Build history of the part. All positions in model axes, mm. Face numbers are marked on the shaded views. Coordinates: 2 decimals unless noted, no trailing zeros. Order: outer loops, then holes, each group sorted by start corner. A loop starts at its lowest first (then second) coordinate and runs counter-clockwise, first axis right, second up. Notation, with made-up numbers: (-35, -18.5) - (-20, -18.5) arc R24 ccw to (-20, 15.5) - close; hole circle Ø9 at (30, -29). An arc over 180 degrees is marked (long way). One line per item, written item: value.
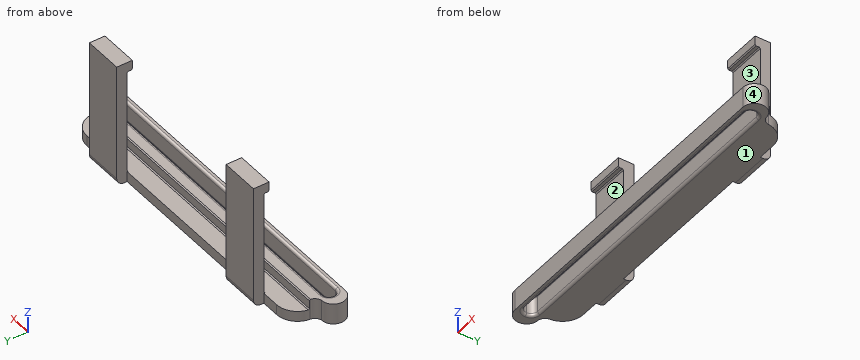
from build123d import *

# Parameters (mm, degrees)
F1_DEPTH    = 8
F2_DEPTH    = 8
F3_DEPTH    = 4
F0_W        = 15
F0_H        = 4
F4_DEPTH    = 48
F5_W        = 15
F5_H        = 3.75
F6_DEPTH    = 2
F7_T1_DEPTH = 43.7732905232
F8_R        = 1
F9_R        = 1
F10_R       = 3
F11_SIZE    = 0.4


# Not quite as in the source:
# - a fillet or chamfer that OpenCascade refuses, or shapes differently, is made with other operations: its cross-section is extruded or revolved along the edge and cut away or added


with BuildPart() as f1:
    # F0 (on Top) → F1 (new body)
    with BuildSketch(Plane.XY):
        with BuildLine():
            Line((60, -5), (-60, -5))
            ThreePointArc((-60, -5), (-61.767766953, -4.267766953), (-62.5, -2.5))
            Line((-62.5, -2.5), (-62.5, -7))
            Line((-62.5, -7), (62.5, -7))
            Line((62.5, -7), (62.5, -2.5))
            ThreePointArc((62.5, -2.5), (61.767766953, -4.267766953), (60, -5))
        make_face()
        with BuildLine():
            Line((62.5, 2), (62.5, -2.5))
            Line((62.5, -2.5), (62.5, -7))
            ThreePointArc((62.5, -7), (67, -2.5), (62.5, 2))
        make_face()
        with BuildLine():
            Line((-62.5, -7), (-62.5, -2.5))
            Line((-62.5, -2.5), (-62.5, 2))
            ThreePointArc((-62.5, 2), (-67, -2.5), (-62.5, -7))
        make_face()
        with BuildLine():
            ThreePointArc((-62.5, -2.5), (-61.767766953, -0.732233047), (-60, 0))
            Line((-60, 0), (60, 0))
            ThreePointArc((60, 0), (61.767766953, -0.732233047), (62.5, -2.5))
            Line((62.5, -2.5), (62.5, 2))
            Line((62.5, 2), (-62.5, 2))
            Line((-62.5, 2), (-62.5, -2.5))
        make_face()
    extrude(amount=F1_DEPTH)

    # F0 (on Top) → F2 (join)
    with BuildSketch(Plane.XY):
        with BuildLine():
            ThreePointArc((-60, 5), (-60.7069250972, 3.047437581), (-62.5, 2))
            Line((-62.5, 2), (62.5, 2))
            ThreePointArc((62.5, 2), (60.7069250972, 3.047437581), (60, 5))
            Line((60, 5), (-60, 5))
        make_face()
    extrude(amount=F2_DEPTH)

    # F0 (on Top) → F3 (join)
    with BuildSketch(Plane.XY):
        Polygon((-60, 12), (-60, 5), (60, 5), (60, 12), (45, 12), (30, 12), (-30, 12), (-45, 12), align=None)
    extrude(amount=F3_DEPTH)

    # F0 (on Top) → F4 (join)
    with BuildSketch(Plane.XY):
        with Locations((-37.5, 14)):
            Rectangle(F0_W, F0_H)
        with Locations((37.5, 14)):
            Rectangle(F0_W, F0_H)
    extrude(amount=F4_DEPTH)

    # F5 (on face) → F6 (join)
    with BuildSketch(Plane.XZ.offset(-12)):
        with Locations((-37.5, 46.125)):
            Rectangle(F5_W, F5_H)
        with Locations((37.5, 46.125)):
            Rectangle(F5_W, F5_H)
    extrude(amount=F6_DEPTH)

    # F7: fillet of radius 8 on 2 edges, made by hand

    # F7_s2 → F7_t1 (cut)
    with BuildSketch(Plane.XY.offset(-19.8866452616)):
        with BuildLine():
            ThreePointArc((52.0453418954, 12), (57.4401609283, 9.9072775118), (60.0125151838, 4.7239819005))
            Line((60.0125151838, 4.7239819005), (60.8092325126, 4.7963800905))
            ThreePointArc((60.8092325126, 4.7963800905), (60.8, 5), (60.8, 12))
            Line((60.8, 12), (60, 12.8))
            Line((60, 12.8), (52.0453418954, 12.8))
            Line((52.0453418954, 12.8), (52.0453418954, 12))
        make_face()
        with BuildLine():
            ThreePointArc((-60.0125151838, 4.7239819005), (-57.4401609283, 9.9072775118), (-52.0453418954, 12))
            Line((-52.0453418954, 12), (-52.0453418954, 12.8))
            Line((-52.0453418954, 12.8), (-60, 12.8))
            Line((-60, 12.8), (-60.8, 12))
            ThreePointArc((-60.8, 12), (-60.8, 5), (-60.8092325126, 4.7963800905))
            Line((-60.8092325126, 4.7963800905), (-60.0125151838, 4.7239819005))
        make_face()
    extrude(amount=F7_T1_DEPTH, mode=Mode.SUBTRACT)

    # F8
    f8_edges = [f1.edges().sort_by_distance(p)[0] for p in [
        (0, 0, 8),
    ]]
    fillet(f8_edges, radius=F8_R)

    # F9
    f9_edges = [f1.edges().sort_by_distance(p)[0] for p in [
        (0, -5, 0),
        (62.5, -2.5, 0),
        (-62.5, -2.5, 0),
        (0, 0, 0),
    ]]
    fillet(f9_edges, radius=F9_R)

    # F10
    f10_edges = [f1.edges().sort_by_distance(p)[0] for p in [
        (-37.5, 16, 0),
        (37.5, 16, 0),
    ]]
    fillet(f10_edges, radius=F10_R)

    # F11
    f11_edges = [f1.edges().sort_by_distance(p)[0] for p in [
        (0, 5, 4),
        (-37.5, 12, 4),
        (37.5, 12, 4),
        (0, 5, 8),
        (37.5, 12, 44.25),
        (-37.5, 12, 44.25),
        (-37.5, 10, 44.25),
        (37.5, 10, 44.25),
    ]]
    chamfer(f11_edges, length=F11_SIZE)


solid = f1.part
1. Two-plate mould, pull along Z, no slides. Class the marked faces 1, 2, 3 and 4: pulls with the +Z half, pulls with the -Z half, needs draft (parallel to the pull), parting line crosses it, or undercut.
Values found:
face 1: pulls with the -Z half
face 2: undercut
face 3: undercut
face 4: needs draft
2. Band-saw the part on B-B, the plane z = 39.5. Give the cut face in (x, y).
Values found:
outline: (-45, 12) - (-30, 12) - (-30, 16) - (-45, 16) - close; (30, 12) - (45, 12) - (45, 16) - (30, 16) - close
3. Probe line 1 along X through (y, z) = (15, 44.5); line 2 along Y through (x, z) = (12, 3.5); line 3 along Y through (x, z) = (-50, 6). List the from-to ranges inside material, lowest first.
Values found:
line 1: x = -45 to -30, 30 to 45
line 2: y = -7 to -5, 0 to 12
line 3: y = -7 to -5, 0 to 5
4. Band-saw the part on C-C, the plane x = -54. Give the cut face in (y, z).
Values found:
outline: (-7, 0) - (-6, 0) arc R1 ccw to (-5, 1) - (-5, 7) arc R1 ccw to (-6, 8) - (-7, 8) - close; (0, 1) arc R1 ccw to (1, 0) - (11.76, 0) - (11.76, 4) - (5.4, 4) - (5, 4.4) - (5, 7.6) - (4.6, 8) - (1, 8) arc R1 ccw to (0, 7) - close
5. Flat gauge pins, fed straight in: P1, Ø6.5, axis at y = 12.5, z = 31, coming from the +X side; P2, Ø3, axis at x = -28, y = 2.5, coming from the +Z side; P3, Ø2.5, axis at x = 40, z = 46.5, coming from the -Y side. Where does each tip first touch, or does it go through?
Values found:
P1: stops at x = 45
P2: stops at z = 8
P3: stops at y = 10
6. Band-saw the part on A-A, the plane x = 39.5. Give the cut face in (y, z), and give its area (3 significant figures).
Values found:
outline: (-7, 0) - (-6, 0) arc R1 ccw to (-5, 1) - (-5, 7) arc R1 ccw to (-6, 8) - (-7, 8) - close; (0, 1) arc R1 ccw to (1, 0) - (13, 0) arc R3 ccw to (16, 3) - (16, 48) - (10, 48) - (10, 44.65) - (10.4, 44.25) - (11.6, 44.25) - (12, 43.85) - (12, 4.4) - (11.6, 4) - (5.4, 4) - (5, 4.4) - (5, 7.6) - (4.6, 8) - (1, 8) arc R1 ccw to (0, 7) - close
area: 281 mm2
